from build123d import *

# Parameters (mm, degrees)
F0_R     = 50
F1_DEPTH = 5
F2_R     = 5
F3_DEPTH = 25


with BuildPart() as f1:
    # F0 (on Top) → F1 (new body, symmetric)
    with BuildSketch(Plane.XY):
        Circle(F0_R)
    extrude(amount=F1_DEPTH, both=True)

    # F2 (on face) → F3 (join)
    with BuildSketch(Plane.XY.offset(5)):
        with Locations((0, 35)):
            Circle(F2_R)
        with Locations((-30.310889, 17.5)):
            Circle(F2_R)
        with Locations((-30.310889, -17.5)):
            Circle(F2_R)
        with Locations((0, -35)):
            Circle(F2_R)
        with Locations((30.310889, -17.5)):
            Circle(F2_R)
        with Locations((30.310889, 17.5)):
            Circle(F2_R)
    extrude(amount=F3_DEPTH)


solid = f1.part
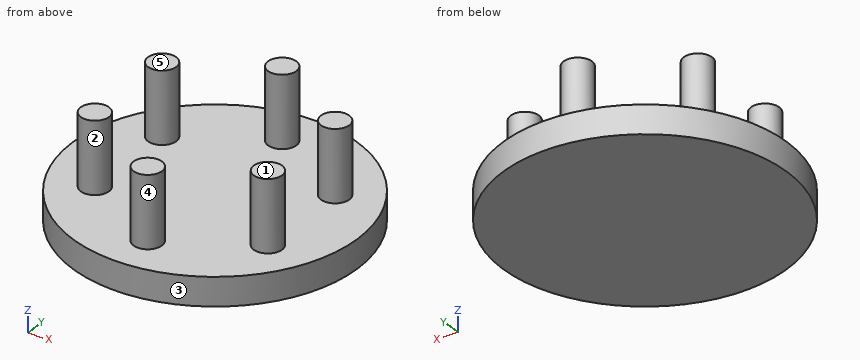
Build history of the part. All positions in model axes, mm. Face numbers are marked on the shaded views. A direction names the side the tool comes from. Round coordinates to 2 decimals unless told otherwise and drop trailing zeros. Order: outer loops, then holes, each group sorted by start corner. A loop starts at its lowest first (then second) coordinate and runs counter-clockwise, first axis right, second up. Notation, with made-up numbers: M -14.5,-6.5 L 6.5,-6.5 A14 ccw 6.5,19.5 Z; hole C 1,37.5 d5. An arc over 180 degrees is marked long. Use CSV: the item, a comma, the result in double quotes. Start each with the question number.
(1) Cut at A-A on z = 25.5. List the corners of the cut face in (x, y).
(2) Tool access for the marked faces 4 and 5: list every direction of +Z, -Z, +X, -X, +Y, -Y with a clear straight run to the whole face (end or side of a thin tool).
(3) Cut at D-D on z = 3. List the corners of the cut face in (x, y), then the cut area to 3 significant figures.
(4) Mould opens along Y. For the marked faces 1, 2 and 3 say: +Y half, -Y half, draft (parallel to the pull), parting line (faces both ways), or undercut.
(5) Flat gauge pins, fed straight in: P1, Ø10, axis at y = -9.5, z = 8, coming from the +X side; P2, Ø1.5, axis at y = -37, z = 13, coming from the +X side; P3, Ø8, axis at x = 11.5, z = 1.5, coming from the +Y side. Where does each tip first touch, or does it go through?
(6) Cut at B-B on x = 0. List the corners of the cut face in (y, z).
(7) Cut at C-C on y = -17.5. List the corners of the cut face in (x, z), then the cut area to 3 significant figures.
(8) Drill centre lines: probe 1 along Y at (x, z) = (-30.5, 11.5); probe 2 along Z at (x, y) = (-35.5, -12); probe 3 along X at (y, z) = (-17, 11). Where is each one in solid material? Low to high.
Findings:
1,outline,"C -30.31,-17.5 d10; C -30.31,17.5 d10; C 0,-35 d10; C 0,35 d10; C 30.31,-17.5 d10; C 30.31,17.5 d10"
2,face 4,"+Z"
2,face 5,"+Z, +X, -X, +Y, -Y"
3,outline,"C 0,0 d100"
3,area,"7,850 mm^2"
4,face 1,"draft"
4,face 2,"undercut"
4,face 3,"parting line"
5,P1,"stops at x = 49.7"
5,P2,"stops at x = 4.84"
5,P3,"stops at y = 49.43"
6,outline,"M -50,-5 L 50,-5 L 50,5 L 40,5 L 40,30 L 30,30 L 30,5 L -30,5 L -30,30 L -40,30 L -40,5 L -50,5 Z"
7,outline,"M -46.84,-5 L 46.84,-5 L 46.84,5 L 35.31,5 L 35.31,30 L 25.31,30 L 25.31,5 L -25.31,5 L -25.31,30 L -35.31,30 L -35.31,5 L -46.84,5 Z"
7,area,"1,440 mm^2"
8,probe 1,"y = -22.5 to -12.5, 12.5 to 22.5"
8,probe 2,"z = -5 to 5"
8,probe 3,"x = -35.29 to -25.34, 25.34 to 35.29"
